Can you work these out from the drawing? Everything is in mm from the part's minimum corner. A direction names the side the tool comes from. Give positions to 0.01 mm unless a question says otherwise; leave off trailing zeros. Write each loop counter-clockwise with the first axis right and the second up, starting at its lowest first coordinate (ties: lowest second). Pieces come first, ordered by that corner, then holes. Notation, with made-up numbers: (-29.75, 27) -> (-5.75, 27) arc R29 cw to (-5.75, 48) -> close; hole circle Ø1 at (28, -18.75). An arc over 180 degrees is marked (long way). Return JSON: item names as keys, results as strings.
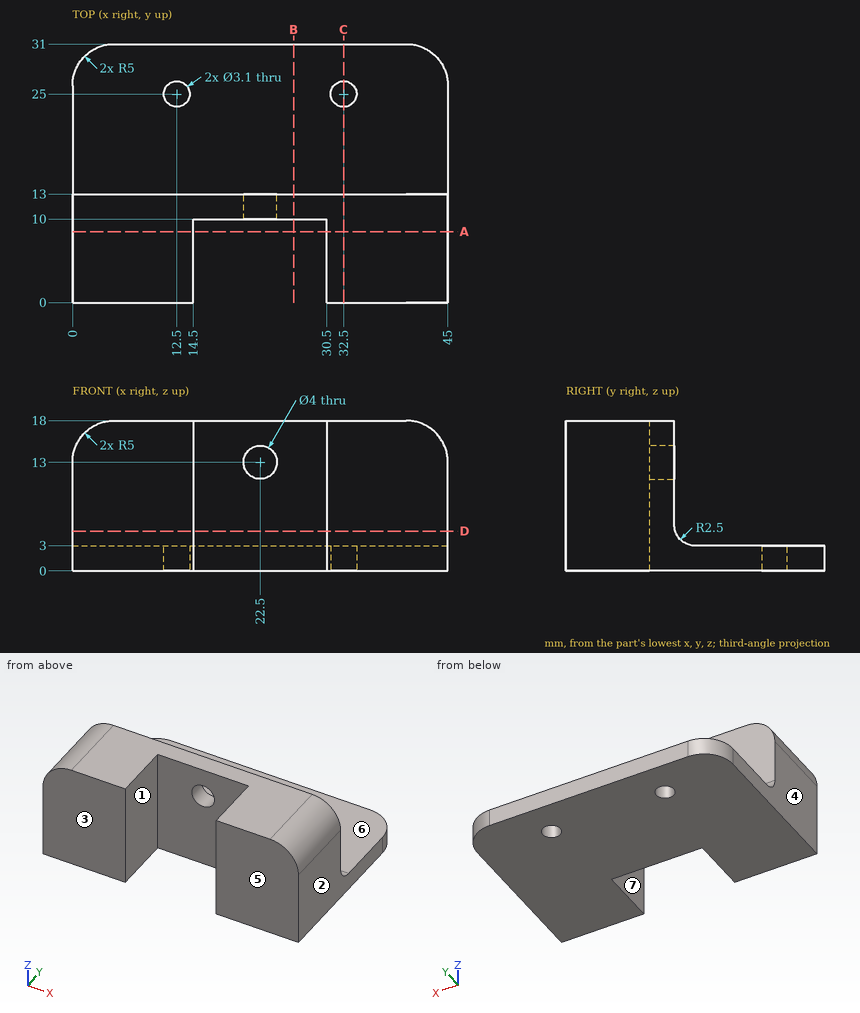
1. Which directions (+Z, -Z, +X, -X, +Y, -Y) give clear straight access to the entire face, cutting with the end or side of a thin tool? Please do the marked faces 5, 6 and 7.
Taken from the geometry:
{"face 5": "+Z, -Z, +X, -X, -Y", "face 6": "+Z, +X, -X, +Y", "face 7": "+Z, -Z, -Y"}
2. Suppose I cut it at A-A, the plane y = 8.5. List the corners of the cut face in (x, z) for me.
Taken from the geometry:
{"outline": "(0, 0) -> (14.5, 0) -> (14.5, 18) -> (5, 18) arc R5 ccw to (0, 13) -> close; (30.5, 0) -> (45, 0) -> (45, 13) arc R5 ccw to (40, 18) -> (30.5, 18) -> close"}
3. If I drill on line 1 (X direction, y = 11.45, z = 13); line 2 (Y direction, x = 32.5, z = 1.3); line 3 (Z direction, x = 42, y = 24.5), over which ranges is the centre line in solid material (lowest first)? Write a range as [from, to].
Taken from the geometry:
{"line 1": "x = [0, 20.5], [24.5, 45]", "line 2": "y = [0, 23.45], [26.55, 31]", "line 3": "z = [0, 3]"}
4. For pin 1 Ø10 at (x, z) = (13.5, 9) entering from +Y; pin 2 Ø3 at (x, z) = (20, 11.5) entering from +Y; pin 3 Ø8 at (x, y) = (5.5, 18) entering from +Z, each with a flat end and sliding along its axis, tell me the tip position at first contact or that it passes through.
Taken from the geometry:
{"pin 1": "stops at y = 13.5", "pin 2": "stops at y = 13", "pin 3": "stops at z = 3.5"}
5. Suppose I cut it at B-B, the plane x = 26.5. List the corners of the cut face in (y, z) for me.
Taken from the geometry:
{"outline": "(10, 0) -> (31, 0) -> (31, 3) -> (15.5, 3) arc R2.5 cw to (13, 5.5) -> (13, 18) -> (10, 18) -> close"}
6. Suppose I cut it at D-D, the plane z = 4.75. List the corners of the cut face in (x, y) for me, and give its area (3 significant figures).
Taken from the geometry:
{"outline": "(0, 0) -> (14.5, 0) -> (14.5, 10) -> (30.5, 10) -> (30.5, 0) -> (45, 0) -> (45, 13.12) -> (0, 13.12) -> close", "area": "430 mm²"}
7. If we mould it in two halves opening along X, with no side actions, what happens to the marked faces 1, 2, 3 and 4? For each: released by +X, released by -X, zero draft, split by the parting line, or undercut.
Taken from the geometry:
{"face 1": "undercut", "face 2": "released by +X", "face 3": "zero draft", "face 4": "released by -X"}
8. Suppose I cut it at C-C, the plane x = 32.5. List the corners of the cut face in (y, z) for me, and give its area (3 significant figures).
Taken from the geometry:
{"outline": "(0, 0) -> (23.45, 0) -> (23.45, 3) -> (15.5, 3) arc R2.5 cw to (13, 5.5) -> (13, 18) -> (0, 18) -> close; (26.55, 0) -> (31, 0) -> (31, 3) -> (26.55, 3) -> close", "area": "280 mm²"}
